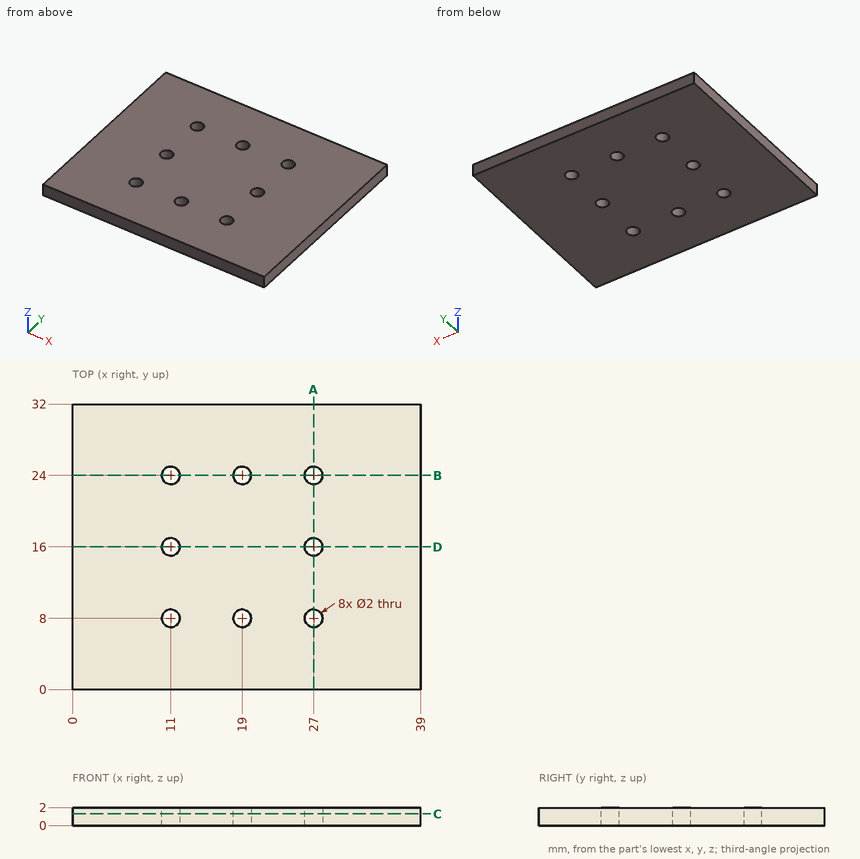
Geometry: see drawing. Coordinates: mm, zero at the bounding-box minimum. Give positions to 0.01 mm unless a question says otherwise; leave off trailing zeros. Order: outer loops, then holes, each group sorted by start corner. A loop starts at its lowest first (then second) coordinate and runs counter-clockwise, first axis right, second up. Notation, with made-up numbers: (51, 57) - (83, 57) arc R34 cw to (83, 87) - close; hole circle Ø1 at (52.5, 47.5). An arc over 180 degrees is marked (long way). Use CSV: the item, a comma, the result in double quotes.
1. Section query D-D (y = 16). Output: boundary loops of the cut face in (x, z).
Answers below:
outline,"(0, 0) - (10, 0) - (10, 2) - (0, 2) - close; (12, 0) - (26, 0) - (26, 2) - (12, 2) - close; (28, 0) - (39, 0) - (39, 2) - (28, 2) - close"
2. Section query C-C (z = 1.3). Give the number of separate pieces and of enclosed holes in the cut face, plus the area to 3 significant figures.
Answers below:
separate pieces,"1"
enclosed holes,"8"
area,"1,220 mm2"
3. Contact query for a flat-ended pin moving along its axis: pin 1 (1.2 mm diameter, centred on x = 19, y = 24, fed in from +Z). Output: stop coordinate, or through.
Answers below:
pin 1,"through"
4. Section query B-B (y = 24). Output: boundary loops of the cut face in (x, z), plus the area to 3 significant figures.
Answers below:
outline,"(0, 0) - (10, 0) - (10, 2) - (0, 2) - close; (12, 0) - (18, 0) - (18, 2) - (12, 2) - close; (20, 0) - (26, 0) - (26, 2) - (20, 2) - close; (28, 0) - (39, 0) - (39, 2) - (28, 2) - close"
area,"66.0 mm2"
5. Material intervals for line 1 along Y through (x, z) = (19, 0.7); line 2 along Y through (x, z) = (27, 0.7); line 3 along X through (y, z) = (24, 1.1), sorted ascending. Write a range as from..to.
Answers below:
line 1,"0..7, 9..23, 25..32"
line 2,"0..7, 9..15, 17..23, 25..32"
line 3,"0..10, 12..18, 20..26, 28..39"
6. Section query A-A (x = 27). Output: boundary loops of the cut face in (y, z), plus the area to 3 significant figures.
Answers below:
outline,"(0, 0) - (7, 0) - (7, 2) - (0, 2) - close; (9, 0) - (15, 0) - (15, 2) - (9, 2) - close; (17, 0) - (23, 0) - (23, 2) - (17, 2) - close; (25, 0) - (32, 0) - (32, 2) - (25, 2) - close"
area,"52.0 mm2"
